Autodesk Inventor part; units mm, degrees
sketch "Sketch1" plane through (0, 0, 0) normal (0, 0, 1) x (1, 0, 0)
  line L0 (-20, 20) -> (20, 20)
  line L1 (20, 20) -> (20, -20)
  line L2 (20, -20) -> (-20, -20)
  line L3 (-20, -20) -> (-20, 20)
  line L4 (-20, 20) -> (20, -20) construction
  line L5 (20, 20) -> (-20, -20) construction
  line L6 (23, 23) -> (-23, 23)
  line L7 (-23, 23) -> (-23, -23)
  line L8 (-23, -23) -> (23, -23)
  line L9 (23, -23) -> (23, 23)
  point P0 (0, 0)
  point P1 (0, 0)
  dimension "d0" = 40
  dimension "d1" = 3
extrude "Extrusion1" add sketch "Sketch1" along normal mid plane 250
properties part number "sessao_07_04_001_001" material "Aluminum 6061"
Geometry: final body of the model. Coordinates: model frame, mm. A direction names the side the tool comes from. Give positions to 0.01 mm unless a question says otherwise; leave off trailing zeros. Write each loop counter-clockwise with the first axis right and the second up, starting at its lowest first coordinate (ties: lowest second). Pieces come first, ordered by that corner, then holes. Notation, with made-up numbers: (-33.5, 61.25) -> (12.5, 61.25) arc R18 ccw to (12.5, 88.25) -> close; hole circle Ø1 at (65.25, 26.25). An arc over 180 degrees is marked (long way). Answer in a Markdown table with one row per item.
(1) Set-up query: faces 5 (the flat face through (0, 20, -2)), 6 (the flat face through (-21, 0, 125)). Return all of +Z, -Z, +X, -X, +Y, -Y with unobstructed straight access to the full face (end or side cutting, diameter ignored); none if empty.
Answers below:
| item | result |
|---|---|
| face 5 | +Z, -Z |
| face 6 | +Z, +X, -X, +Y, -Y |
(2) Draft query along Y for faces 1 (the flat face through (-21, 0, -125)), 2 (the flat face through (0, -23, -2)), 3 (the flat face through (0, -20, -2)), 4 (the flat face through (0, 23, -2)). Return one class per face: +Y half, -Y half, draft (parallel to the pull), parting line (faces both ways), or undercut.
Answers below:
| item | result |
|---|---|
| face 1 | draft |
| face 2 | -Y half |
| face 3 | undercut |
| face 4 | +Y half |
(3) Pin query (flat end, axial travel): pin 1 (8 mm diameter, centred on x = 14.5, y = 17, fed in from -Z). Return the tip coordinate at first contact, or that it passes through.
Answers below:
| item | result |
|---|---|
| pin 1 | z = -125 |
(4) Section query B-B on z = 36.5. Return loops of the section in (x, y), then the cut area to 3 significant figures.
Answers below:
| item | result |
|---|---|
| outline | (-23, -23) -> (23, -23) -> (23, 23) -> (-23, 23) -> close; hole (-20, -20) -> (20, -20) -> (20, 20) -> (-20, 20) -> close |
| area | 516 mm^2 |
(5) Ray query, line 1 along Y through (x, z) = (-6, -21). Return the intervals inside material, ascending. Write a range as [from, to].
Answers below:
| item | result |
|---|---|
| line 1 | [-23, -20], [20, 23] |
(6) Section query A-A on y = -17. Return loops of the section in (x, z).
Answers below:
| item | result |
|---|---|
| outline | (-23, -125) -> (-20, -125) -> (-20, 125) -> (-23, 125) -> close; (20, -125) -> (23, -125) -> (23, 125) -> (20, 125) -> close |
